from build123d import *

# Parameters (mm, degrees)
F0_W     = 120
F0_H     = 31
F1_DEPTH = 15
F2_R     = 1.9
F3_DEPTH = 60
F5_DEPTH = 70
F6_R     = 1.9
F7_DEPTH = 80
F9_DEPTH = 70


with BuildPart() as f1:
    # F0 (on Front) → F1 (new body)
    with BuildSketch(Plane.XZ):
        with Locations((-32.620786, -3.705296)):
            Rectangle(F0_W, F0_H)
    extrude(amount=F1_DEPTH)

    # F2 (on face) → F3 (cut)
    with BuildSketch(Plane(origin=(0, 0, -19.205296), x_dir=(1, 0, 0), z_dir=(0, 0, -1))):
        with Locations((21.879214, 7.5)):
            Circle(F2_R)
    extrude(amount=-F3_DEPTH, mode=Mode.SUBTRACT)

    # F4 (on face) → F5 (cut)
    with BuildSketch(Plane(origin=(0, 0, -19.205296), x_dir=(1, 0, 0), z_dir=(0, 0, -1))):
        with BuildLine():
            ThreePointArc((-84.706673, 0), (-92.206673, 7.5), (-84.706673, 15))
            Line((-84.706673, 15), (-92.620786, 15))
            Line((-92.620786, 15), (-92.620786, 0))
            Line((-92.620786, 0), (-84.706673, 0))
        make_face()
    extrude(amount=-F5_DEPTH, mode=Mode.SUBTRACT)

    # F6 (on face) → F7 (cut)
    with BuildSketch(Plane(origin=(0, 0, -19.205296), x_dir=(1, 0, 0), z_dir=(0, 0, -1))):
        with Locations((-86.707558, 7.5987)):
            Circle(F6_R)
    extrude(amount=-F7_DEPTH, mode=Mode.SUBTRACT)

    # F8 (on face) → F9 (cut)
    with BuildSketch(Plane(origin=(0, 0, -19.205296), x_dir=(1, 0, 0), z_dir=(0, 0, -1))):
        with BuildLine():
            ThreePointArc((19.677406, 15), (27.177406, 7.5), (19.677406, 0))
            Line((19.677406, 0), (27.379214, 0))
            Line((27.379214, 0), (27.379214, 15))
            Line((27.379214, 15), (19.677406, 15))
        make_face()
    extrude(amount=-F9_DEPTH, mode=Mode.SUBTRACT)


solid = f1.part
For this review, take the finished solid that the model builds, in its own axes (mm). Round coordinates to 2 decimals unless told otherwise and drop trailing zeros. Loops run counter-clockwise (first coordinate to the right, second up) from the corner with the lowest first, then second, coordinate; pieces in that order, holes last. Notation, with made-up numbers: (77.5, 36) - (103.5, 36) arc R26 cw to (103.5, 72) - close; hole circle Ø11 at (27.25, 6). An arc over 180 degrees is marked (long way). One line per item, written item: value. Start each with the question number.
Item 1: For L1, parallel to X at y = -7.5, z = 2 (3 decimals); L2, parallel to X at y = -6, z = 1.5; L3, parallel to Y at x = -86.5, z = -0.5, list the stretches that pass through material, from the lowest coordinate up.
Item 2: Take a section at A-A (z = 4). Give the boundary of the cut face in (x, y).
Item 3: Clearance check with flat-ended pins moving along their axes: pin 1 Ø3 at (y, z) = (-10.5, 7) entering from +X; pin 2 Ø3 at (x, y) = (21.88, -7.5) entering from +Z; pin 3 Ø1.5 at (y, z) = (-12, -4) entering from +X; pin 4 Ø1.5 at (y, z) = (-10.5, -16) entering from -X. State where each tip first meets the part, or that it passes through.
Item 4: Take a section at B-B (y = -11.75). Give the boundary of the cut face in (x, z).
Answer below:
1. L1: x = -92.207 to -88.605, -84.81 to 19.979, 23.779 to 27.177
1. L2: x = -92.06 to -87.73, -85.68 to 20.71, 23.05 to 27.03
1. L3: y = -14.78 to -9.49, -5.71 to -0.22
2. outline: (-84.71, -15) - (19.68, -15) arc R7.5 ccw to (19.68, 0) - (-84.71, 0) arc R7.5 ccw to start; hole circle Ø3.8 at (-86.71, -7.6); hole circle Ø3.8 at (21.88, -7.5)
3. pin 1: stops at x = 27.03
3. pin 2: passes through
3. pin 3: stops at x = 26.17
3. pin 4: stops at x = -91.86
4. outline: (-90.89, -19.21) - (25.86, -19.21) - (25.86, 11.79) - (-90.89, 11.79) - close
